from build123d import *

# Parameters (mm, degrees)
SKETCH_1_W      = 25
SKETCH_1_H      = 24
SKETCH_1_R      = 1
EXTRUDE_1_DEPTH = 1
SKETCH_2_R      = 1.75
EXTRUDE_2_DEPTH = 1
FILLET_1_R      = 0.2
SKETCH_3_W      = 20.5
SKETCH_3_H      = 4
EXTRUDE_3_DEPTH = 2.7
SKETCH_4_R      = 8
EXTRUDE_4_DEPTH = 12
SKETCH_5_R      = 7
EXTRUDE_5_DEPTH = 2
FILLET_2_R      = 0.3


with BuildPart() as part:
    # Эскиз1 → Бобышка-Вытянуть1 (new body)
    with BuildSketch(Plane(origin=(0, 0, 0), x_dir=(1, 0, 0), z_dir=(0, 1, 0))):
        Rectangle(SKETCH_1_W, SKETCH_1_H)
        with Locations((-10.5, 10)):
            Circle(SKETCH_1_R, mode=Mode.SUBTRACT)
        with Locations((10.5, 10)):
            Circle(SKETCH_1_R, mode=Mode.SUBTRACT)
        with Locations((10.5, -4)):
            Circle(SKETCH_1_R, mode=Mode.SUBTRACT)
        with Locations((-10.5, -4)):
            Circle(SKETCH_1_R, mode=Mode.SUBTRACT)
    extrude(amount=EXTRUDE_1_DEPTH)

    # Эскиз2 → Бобышка-Вытянуть2 (add)
    with BuildSketch(Plane(origin=(0, 1, 0), x_dir=(1, 0, 0), z_dir=(0, 1, 0))):
        with Locations((-9, 3.5)):
            Circle(SKETCH_2_R)
        with Locations((9, 3.5)):
            Circle(SKETCH_2_R)
    extrude(amount=EXTRUDE_2_DEPTH)

    # Скругление1
    fillet_1_edges = [part.edges().sort_by_distance(p)[0] for p in [
        (-10.75, 1, -3.5),
        (-10.75, 2, -3.5),
        (7.25, 1, -3.5),
        (7.25, 2, -3.5),
    ]]
    fillet(fillet_1_edges, radius=FILLET_1_R)

    # Эскиз3 → Бобышка-Вытянуть3 (add)
    with BuildSketch(Plane.XZ):
        with Locations((0, 8.5)):
            Rectangle(SKETCH_3_W, SKETCH_3_H)
        Polygon((-11, 10.5), (-10.25, 10.5), (10.25, 10.5), (11, 10.5), (11, 12), (-11, 12), align=None)
    extrude(amount=EXTRUDE_3_DEPTH)

    # Эскиз4 → Бобышка-Вытянуть4 (add)
    with BuildSketch(Plane.XZ):
        with Locations((0, -3)):
            Circle(SKETCH_4_R)
    extrude(amount=EXTRUDE_4_DEPTH)

    # Эскиз5 → Бобышка-Вытянуть5 (add)
    with BuildSketch(Plane.XZ.offset(12)):
        with Locations((0, -3)):
            Circle(SKETCH_5_R)
    extrude(amount=EXTRUDE_5_DEPTH)

    # Скругление2
    fillet_2_edges = [part.edges().sort_by_distance(p)[0] for p in [
        (-7, -14, -3),
    ]]
    fillet(fillet_2_edges, radius=FILLET_2_R)


solid = part.part
Verification items for the finished model (mm, model axes). A direction names the side the tool comes from. Round coordinates to 2 decimals unless told otherwise and drop trailing zeros. Loops run counter-clockwise (first coordinate to the right, second up) from the corner with the lowest first, then second, coordinate; pieces in that order, holes last. Notation, with made-up numbers: M -3,41.25 L 7,41.25 A15 cw 7,67.25 Z; hole C 24,56 d8. An arc over 180 degrees is marked long. Write each question's results on one line, items separated by ' | '.
1) Scan lines: L1, parallel to X at y = 0.8, z = 4; L2, parallel to Z at x = -10.5, y = 0.6; L3, parallel to Y at x = -7.5, z = 6.75. Record each from-to range of solid material in increasing order. Write a range as from..to.
Checks:
L1: x = -12.5..-11.5, -9.5..9.5, 11.5..12.5 | L2: z = -12..-11, -9..3, 5..12 | L3: y = -2.7..1
2) Section check C-C on y = -12.5. Record the boundary of the cut face in (x, z), then the cut area to 3 significant figures.
Checks:
outline: C 0,-3 d14 | area: 154 mm2
3) Mould release check, pull along X, two halves, no side actions. Record for faces 5 (the cylindrical face through (-10.63, 0.49, -10.99)), 6 (the flat face through (12.5, 0.5, 0.2)), 7 (the flat face through (-10.25, -1, 8)): released by +X, released by -X, zero draft, split by the parting line, or undercut.
Checks:
face 5: undercut | face 6: released by +X | face 7: released by -X
4) Access from +Z, -Z, +X, -X, +Y, -Y to the whole of each face (thin tool, end or side, straight path). Record for faces 1 (the flat face through (10.25, -1, 8)), 2 (the flat face through (-11, -1, 11)), 3 (the cylindrical face through (9.81, 1.5, -1.95)), 4 (the flat face through (4, -12, -9)).
Checks:
face 1: -Z, +X, -Y | face 2: +Z, -Z, -X, -Y | face 3: +Y | face 4: -Y
5) Gauge pin test, flat ends, axial feed: P1, Ø4, axis at y = -9.5, z = 0, coming from the -X side; P2, Ø1.6, axis at x = 2, z = 10, coming from the -Y side; P3, Ø2, axis at x = 4, y = -6.5, coming from the +Z side; P4, Ø1.8, axis at x = 10.5, z = 4, coming from the +Y side. Record the tip position at first contact, or that the pin passes through.
Checks:
P1: stops at x = -7.94 | P2: stops at y = -2.7 | P3: stops at z = 4.42 | P4: passes through
6) Section check A-A on y = -1.25. Record the boundary of the cut face in (x, z).
Checks:
outline: M -11,10.5 L -10.25,10.5 L -10.25,6.5 L 10.25,6.5 L 10.25,10.5 L 11,10.5 L 11,12 L -11,12 Z; C 0,-3 d16
7) Section check B-B on z = 9.5. Record the boundary of the cut face in (x, y), then the cut area to 4 significant figures.
Checks:
outline: M -12.5,0 L -10.25,0 L -10.25,-2.7 L 10.25,-2.7 L 10.25,0 L 12.5,0 L 12.5,1 L -12.5,1 Z | area: 80.35 mm2
